The figure shows three views and two pictorial views of one solid part (mm, origin at its lowest corner). Answer the questions. Coordinates: 2 decimals unless noted, no trailing zeros. Order: outer loops, then holes, each group sorted by start corner. A loop starts at its lowest first (then second) coordinate and runs counter-clockwise, first axis right, second up. Notation, with made-up numbers: M 20.25,81 L 62.25,81 A29 ccw 62.25,112 Z; hole C 70,44 d8. An arc over 180 degrees is marked long. Write item = value, one per line. Start each with the question number.
Q1. Find section C-C on z = 48.5. Give the vertices of the cut face in (x, y), and give its area (3 significant figures).
Q2. Each of these flat-tipped pins is pushed along its axis until it touches: P1, Ø8, axis at x = 216, z = 99.5, coming from the -Y side; P2, Ø12, axis at y = 37, z = 109, coming from the +X side. Where does it stop, or does it pass through?
Q3. Determine the mould class of the marked faces 1 and 2 for opening direction Z: released by +Z, released by -Z, zero draft, split by the parting line, or undercut.
Q4. Straight lines are drawn through the part: line 1 along Y through (x, z) = (247.5, 122); line 2 along X through (y, z) = (60, 37.5); line 3 along X through (y, z) = (7.5, 114.5) (1 decimal). For each, find the intervals that lie inside material, in ascending order.
Q5. Find section A-A on x = 33. Give the vertices of the cut face in (y, z), and give its area (3 significant figures).
Q6. Find section D-D on x = 181.5. Give the vertices of the cut face in (y, z) (1 decimal).
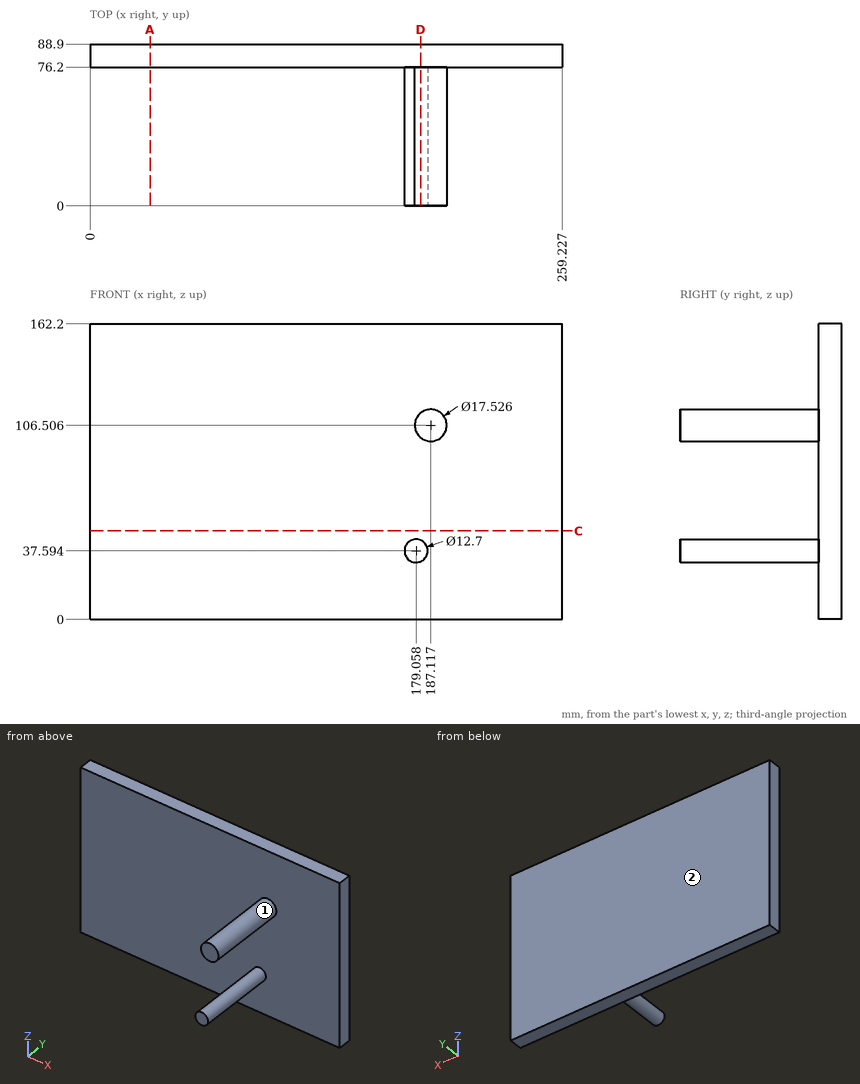
Findings below:
q1.outline = M 0,76.2 L 259.23,76.2 L 259.23,88.9 L 0,88.9 Z
q1.area = 3,290 mm^2
q2.P1 = 76.2
q2.P2 = 195.88
q3.face_1 = undercut
q3.face_2 = zero draft
q4.line_1 = 76.2 to 88.9
q4.line_2 = 172.71 to 185.41
q4.line_3 = 183.5 to 190.7
q5.outline = M 76.2,0 L 88.9,0 L 88.9,162.2 L 76.2,162.2 Z
q5.area = 2,060 mm^2
q6.outline = M 0,31.7 L 76.2,31.7 L 76.2,0 L 88.9,0 L 88.9,162.2 L 76.2,162.2 L 76.2,113.2 L 0,113.2 L 0,99.8 L 76.2,99.8 L 76.2,43.5 L 0,43.5 Z
